Design review of the part built by this model. Coordinates are the model's own, in mm. Face numbers are marked on the shaded views. Round coordinates to 2 decimals unless told otherwise and drop trailing zeros. Order: outer loops, then holes, each group sorted by start corner. A loop starts at its lowest first (then second) coordinate and runs counter-clockwise, first axis right, second up.
from build123d import *

# Parameters (mm, degrees)
ESBO_O2_W                  = 42.5
ESBO_O2_H                  = 42.5
RESSALTO_EXTRUS_O1_DEPTH   = 20
RESSALTO_EXTRUS_O1_2_DEPTH = 20
RESSALTO_EXTRUS_O1_3_DEPTH = 20
RESSALTO_EXTRUS_O1_4_DEPTH = 20
RESSALTO_EXTRUS_O2_DEPTH   = 15


with BuildPart() as part:
    # Esbo_o2 → Ressalto-extrus_o1 (new body)
    with BuildSketch(Plane(origin=(0, 0, 0), x_dir=(1, 0, 0), z_dir=(0, 1, 0))):
        with Locations((-28.75, 28.75)):
            Rectangle(ESBO_O2_W, ESBO_O2_H)
    extrude(amount=RESSALTO_EXTRUS_O1_DEPTH)



with BuildPart() as body_2:
    # Esbo_o2 → Ressalto-extrus_o1 2 (new body)
    with BuildSketch(Plane(origin=(0, 0, 0), x_dir=(1, 0, 0), z_dir=(0, 1, 0))):
        with Locations((28.75, 28.75)):
            Rectangle(ESBO_O2_W, ESBO_O2_H)
    extrude(amount=RESSALTO_EXTRUS_O1_2_DEPTH)


with BuildPart() as body_3:
    # Esbo_o2 → Ressalto-extrus_o1 3 (new body)
    with BuildSketch(Plane(origin=(0, 0, 0), x_dir=(1, 0, 0), z_dir=(0, 1, 0))):
        with Locations((-28.75, -28.75)):
            Rectangle(ESBO_O2_W, ESBO_O2_H)
    extrude(amount=RESSALTO_EXTRUS_O1_3_DEPTH)


with BuildPart() as body_4:
    # Esbo_o2 → Ressalto-extrus_o1 4 (new body)
    with BuildSketch(Plane(origin=(0, 0, 0), x_dir=(1, 0, 0), z_dir=(0, 1, 0))):
        with Locations((28.75, -28.75)):
            Rectangle(ESBO_O2_W, ESBO_O2_H)
    extrude(amount=RESSALTO_EXTRUS_O1_4_DEPTH)


with BuildPart() as part_1:
    add(part.part)

    add(body_2.part)  # Ressalto-extrus_o2 merges body 2

    add(body_3.part)  # Ressalto-extrus_o2 merges body 3

    add(body_4.part)  # Ressalto-extrus_o2 merges body 4
    # Esbo_o2_3 → Ressalto-extrus_o2 (add)
    with BuildSketch(Plane(origin=(0, 0, 0), x_dir=(1, 0, 0), z_dir=(0, 1, 0))):
        Polygon((50, 7.5), (7.5, 7.5), (7.5, 50), (-7.5, 50), (-7.5, 7.5), (-50, 7.5), (-50, -7.5), (-7.5, -7.5), (-7.5, -50), (7.5, -50), (7.5, -7.5), (50, -7.5), align=None)
    extrude(amount=RESSALTO_EXTRUS_O2_DEPTH)


solid = part_1.part
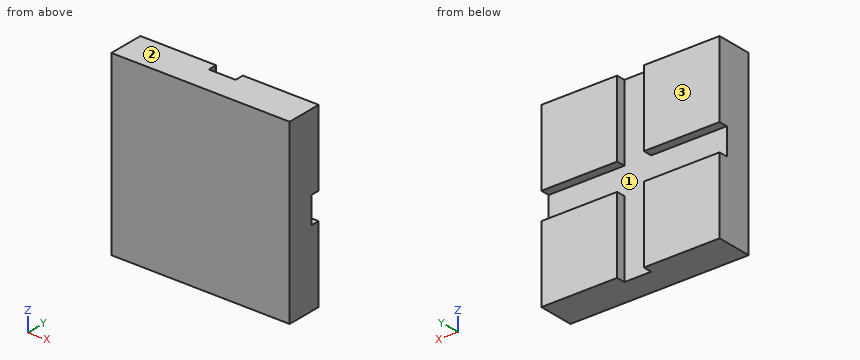
1) Take a section at B-B on x = 13.5. Give the boundary of the cut face in (y, z), plus the area to 4 significant figures.
Results:
outline: (0, -50) - (20, -50) - (20, -7.5) - (15, -7.5) - (15, 7.5) - (20, 7.5) - (20, 50) - (0, 50) - close
area: 1,925 mm2
2) Clearance check with a flat-ended pin moving along its axis: P1, Ø1.5, axis at x = 2.5, y = 16, coming from the -Z side. State where the tip first meets the part, or that it passes through.
Results:
P1: passes through
3) To check wall thickness, follow line 1 along X through (y, z) = (19, -30); line 2 along Y through (x, z) = (-45, 1). State the ranges of each line that lie inside material, in increasing order.
Results:
line 1: x = -50 to -7.5, 7.5 to 50
line 2: y = 0 to 15
4) The part is to be moulded in two halves that separate along Z. For the marked faces 1, 2 and 3, say which applies: released by +Z, released by -Z, zero draft, split by the parting line, or undercut.
Results:
face 1: undercut
face 2: released by +Z
face 3: zero draft
5) Take a section at C-C on y = 16.75. Give the boundary of the cut face in (x, z), plus the area to 4 significant figures.
Results:
outline: (-50, -50) - (-7.5, -50) - (-7.5, -7.5) - (-50, -7.5) - close; (-50, 7.5) - (-7.5, 7.5) - (-7.5, 50) - (-50, 50) - close; (7.5, -50) - (50, -50) - (50, -7.5) - (7.5, -7.5) - close; (7.5, 7.5) - (50, 7.5) - (50, 50) - (7.5, 50) - close
area: 7,225 mm2
6) Take a section at A-A on z = 12. Give the boundary of the cut face in (x, y).
Results:
outline: (-50, 0) - (50, 0) - (50, 20) - (7.5, 20) - (7.5, 15) - (-7.5, 15) - (-7.5, 20) - (-50, 20) - close
